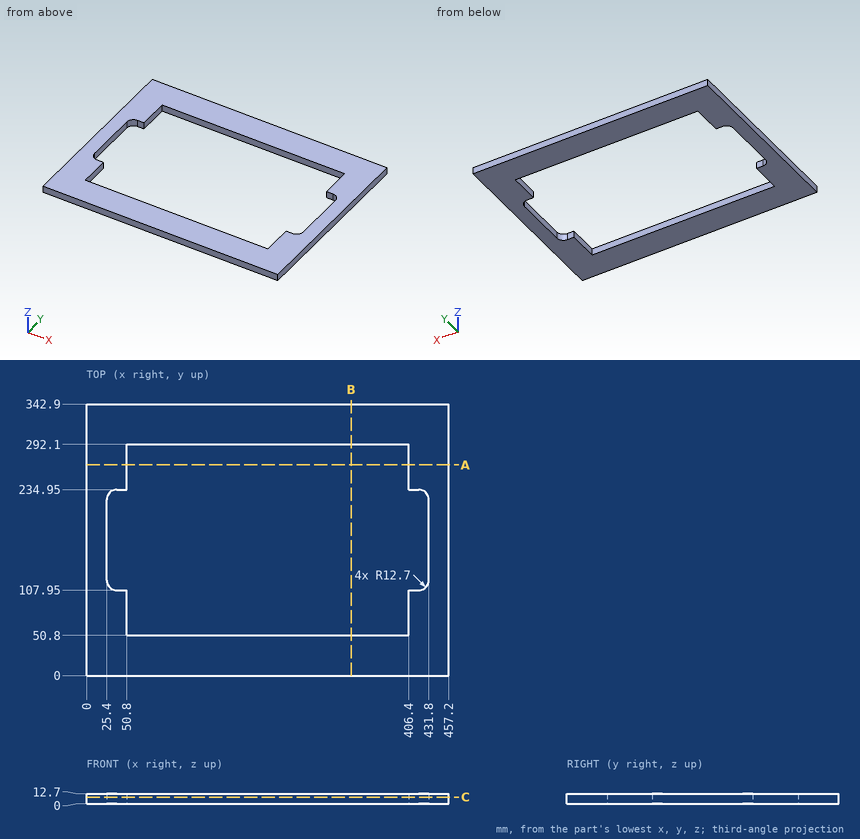
Drawing for the job (mm, zero at the part's lowest x, y, z). Round coordinates to 2 decimals unless told otherwise and drop trailing zeros. Order: outer loops, then holes, each group sorted by start corner. A loop starts at its lowest first (then second) coordinate and runs counter-clockwise, first axis right, second up. Notation, with made-up numbers: (44, 82.25) -> (61, 82.25) arc R7 ccw to (61, 86.25) -> close; hole circle Ø10 at (29.25, 28.5). An arc over 180 degrees is marked (long way). Put each result on its own line as item: value.
Q1. Wall check: line 1 (X direction, y = 182.5, z = 7.25); line 2 (Y direction, x = 281, z = 5); line 3 (X direction, y = 267, z = 4). Give the ranges that are in metal, low to high. Write a range as [from, to].
From the geometry:
line 1: x = [0, 25.4], [431.8, 457.2]
line 2: y = [0, 50.8], [292.1, 342.9]
line 3: x = [0, 50.8], [406.4, 457.2]
Q2. Band-saw the part on A-A (y = 266). Give the cut face in (x, z).
From the geometry:
outline: (0, 0) -> (50.8, 0) -> (50.8, 12.7) -> (0, 12.7) -> close; (406.4, 0) -> (457.2, 0) -> (457.2, 12.7) -> (406.4, 12.7) -> close
Q3. Band-saw the part on C-C (z = 8.25). Give the cut face in (x, y).
From the geometry:
outline: (0, 0) -> (457.2, 0) -> (457.2, 342.9) -> (0, 342.9) -> close; hole (25.4, 120.65) arc R12.7 ccw to (38.1, 107.95) -> (50.8, 107.95) -> (50.8, 50.8) -> (406.4, 50.8) -> (406.4, 107.95) -> (419.1, 107.95) arc R12.7 ccw to (431.8, 120.65) -> (431.8, 222.25) arc R12.7 ccw to (419.1, 234.95) -> (406.4, 234.95) -> (406.4, 292.1) -> (50.8, 292.1) -> (50.8, 234.95) -> (38.1, 234.95) arc R12.7 ccw to (25.4, 222.25) -> close
Q4. Band-saw the part on B-B (x = 334). Give the cut face in (y, z).
From the geometry:
outline: (0, 0) -> (50.8, 0) -> (50.8, 12.7) -> (0, 12.7) -> close; (292.1, 0) -> (342.9, 0) -> (342.9, 12.7) -> (292.1, 12.7) -> close
